Could you check a few things on this model? Use its own coordinates, in mm. Round coordinates to 2 decimals unless told otherwise and drop trailing zeros. Write each loop counter-clockwise with the first axis right and the second up, starting at its lowest first coordinate (ties: lowest second). Pieces come first, ordered by that corner, then holes.
```python
from build123d import *

# Parameters (mm, degrees)
SKETCH_2_R          = 100
CUT_EXTRUDE_1_DEPTH = 101


with BuildPart() as part:
    # 草图1 → 旋转7 (revolve)
    with BuildSketch(Plane.XY):
        with BuildLine():
            Line((0, 100), (0, -100))
            ThreePointArc((0, -100), (100, 0), (0, 100))
        make_face()
    revolve(axis=Axis((0, 100, 0), (0, -1, 0)))

    # 草图3 → 切除-旋转1 (revolve, cut)
    with BuildSketch(Plane.XY):
        with BuildLine():
            Line((0, 98), (0, -98))
            ThreePointArc((0, -98), (98, 0), (0, 98))
        make_face()
    revolve(axis=Axis((0, 98, 0), (0, -1, 0)), mode=Mode.SUBTRACT)

    # 草图2 → 切除-拉伸1 (cut, through all)
    with BuildSketch(Plane.XY):
        Circle(SKETCH_2_R)
    extrude(amount=CUT_EXTRUDE_1_DEPTH, mode=Mode.SUBTRACT)


solid = part.part
```
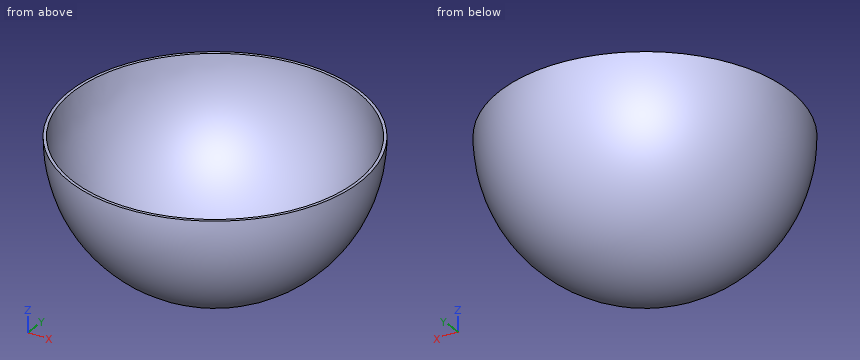
Q1. If I drill on L1, parallel to Y at x = 47.5, z = -75.5; L2, parallel to Y at x = 32.5, z = -82; L3, parallel to X at y = 70, z = -57, over which ranges is the centre line in solid material (lowest first)?
Q2. Imagine slicing it at B-B, the plane x = -13.5. Write out the boundary of the cut face in (y, z).
Q3. I'm going to push flat-ended pins straight in: pin 1 Ø1.5 at (y, z) = (62.5, -56.5) entering from +X; pin 2 Ø6 at (x, z) = (16, -39.5) entering from -Y; pin 3 Ø1 at (x, y) = (-48, -51) entering from +Z. Where does each tip first touch, or does it pass through?
Q4. Imagine slicing it at C-C, the plane y = 63. Write out the boundary of the cut face in (x, z), then the cut area to 3 significant figures.
Q5. Imagine slicing it at A-A, the plane z = -71. Write out the boundary of the cut face in (x, y), then the cut area to 3 significant figures.
Results found:
1. L1: y = -45.21 to -40.59, 40.59 to 45.21
1. L2: y = -47.11 to -42.71, 42.71 to 47.11
1. L3: x = -43.02 to -38.14, 38.14 to 43.02
2. outline: (-99.08, 0) arc R99.08 ccw to (99.08, 0) - (97.07, 0) arc R97.07 cw to (-97.07, 0) - close
3. pin 1: stops at x = 55.02
3. pin 2: stops at y = -91.82
3. pin 3: stops at z = -68.03
4. outline: (-77.66, 0) arc R77.66 ccw to (77.66, 0) - (75.07, 0) arc R75.07 cw to (-75.07, 0) - close
4. area: 622 mm2
5. outline: circle Ø140.84 at (0, 0); hole circle Ø135.1 at (0, 0)
5. area: 1,240 mm2
